Check sheet for the modelled part. Datum: model origin and axes. Units: mm. Face numbers are marked on the shaded views. Coordinates: 2 decimals unless noted, no trailing zeros. Write each loop counter-clockwise with the first axis right and the second up, starting at its lowest first coordinate (ties: lowest second). Pieces come first, ordered by that corner, then holes. Notation, with made-up numbers: (73, 12) -> (101, 12) arc R20 cw to (101, 31) -> close; hole circle Ø1 at (77.25, -11.5). An arc over 180 degrees is marked (long way). One line per item, written item: value. Start each with the question number.
1) Sectioned sample at C-C on y = -5.5. Enter the section's corners in (x, z), plus the area to 3 significant figures.
2) Sectioned sample at A-A on z = -6.75. Enter the section's corners in (x, y).
3) Sectioned sample at B-B on y = 2.25. Enter the section's corners in (x, z).
4) Scan lines: line 1 along Z through (x, y) = (-4.25, 5.5); line 2 along Y through (x, z) = (9.25, 5.25). Record each from-to range of solid material in increasing order. Write a range as [from, to].
5) Draft check along Y on the marked faces 1, 2 and 3. Enter one of: +Y half, -Y half, draft (parallel to the pull), parting line (faces both ways), or undercut.
6) Gauge pin test, flat end, axial feed: P1, Ø1, axis at x = -1.5, y = 2, coming from the +Z side. Record the tip position at first contact, or that the pin passes through.
7) Sectioned sample at D-D on z = 0.75. Enter the section's corners in (x, y).
Autodesk Inventor part; units mm, degrees
ref_plane "YZ Plane" through (0, 0, 0) normal (1, 0, 0) x (0, 1, 0)
ref_plane "XZ Plane" through (0, 0, 0) normal (0, 1, 0) x (-1, 0, 0)
ref_plane "XY Plane" through (0, 0, 0) normal (0, 0, 1) x (1, 0, 0)
sketch "Esboço1" plane through (0, 0, 0) normal (0, 0, 1) x (1, 0, 0)
  line L0 (-10, -10) -> (10, -10)
  line L1 (10, -10) -> (10, 10)
  line L2 (10, 10) -> (-10, 10)
  line L3 (-10, 10) -> (-10, -10)
  line L4 (-10, -10) -> (10, 10) construction
  line L5 (10, -10) -> (-10, 10) construction
  point P0 (0, 0)
  dimension "d0" = 20
  dimension "d1" = 20
extrude "Extrusão1" add sketch "Esboço1" along normal mid plane 20
sketch "Esboço2" plane through (0, 0, 10) normal (0, 0, 1) x (1, 0, 0)
  line L0 (-10, 10) -> (10, 10) construction
  line L1 (10, 10) -> (10, -10) construction
  line L2 (10, -10) -> (-10, -10) construction
  line L3 (-10, -10) -> (-10, 10) construction
  line L4 (5.9015, -7.5) -> (3.6163, -7.5)
  line L5 (3.6163, -7.5) -> (-0.0304, -1.5194)
  line L6 (-0.0304, -1.5194) -> (-3.75, -7.5)
  line L7 (-3.75, -7.5) -> (-5.9015, -7.5)
  line L8 (-5.9015, -7.5) -> (-1.1244, 0.0122)
  line L9 (-1.1244, 0.0122) -> (-5.7557, 7.5)
  line L10 (-5.7557, 7.5) -> (-3.4704, 7.5)
  line L11 (-3.4704, 7.5) -> (0.1033, 1.6288)
  line L12 (0.1033, 1.6288) -> (3.75, 7.5)
  line L13 (3.75, 7.5) -> (5.9015, 7.5)
  line L14 (5.9015, 7.5) -> (1.2095, 0.1094)
  line L15 (1.2095, 0.1094) -> (5.9015, -7.5)
  point P0 (0, 0)
extrude "Extrusão2" cut sketch "Esboço2" against normal blind 1
sketch "Esboço3" plane through (10, -10, 10) normal (1, 0, 0) x (0, 0, -1)
  line L0 (0, 20) -> (20, 20) construction
  line L1 (20, 20) -> (20, 0) construction
  line L2 (20, 0) -> (0, 0) construction
  line L3 (0, 0) -> (0, 20) construction
  line L4 (15.9562, 17.5) -> (10.8874, 9.137)
  line L5 (10.8874, 9.137) -> (10.8874, 2.5)
  line L6 (10.8874, 2.5) -> (8.8938, 2.5)
  line L7 (8.8938, 2.5) -> (8.8938, 8.9303)
  line L8 (8.8938, 8.9303) -> (3.825, 17.5)
  line L9 (3.825, 17.5) -> (6.0373, 17.5)
  line L10 (6.0373, 17.5) -> (9.9028, 10.8995)
  line L11 (9.9028, 10.8995) -> (13.8412, 17.5)
  line L12 (13.8412, 17.5) -> (15.9562, 17.5)
  point P0 (10, 10)
extrude "Extrusão3" cut sketch "Esboço3" against normal blind 1
sketch "Esboço4" plane through (-10, 10, 10) normal (0, 1, 0) x (1, 0, 0)
  line L0 (0, 20) -> (20, 20) construction
  line L1 (20, 20) -> (20, 0) construction
  line L2 (20, 0) -> (0, 0) construction
  line L3 (0, 0) -> (0, 20) construction
  line L4 (15.3181, 2.5) -> (4.84, 2.5)
  line L5 (4.84, 2.5) -> (4.84, 4.3598)
  line L6 (4.84, 4.3598) -> (12.8626, 15.7253)
  line L7 (12.8626, 15.7253) -> (5.2046, 15.7253)
  line L8 (5.2046, 15.7253) -> (5.2046, 17.5)
  line L9 (5.2046, 17.5) -> (15.1114, 17.5)
  line L10 (15.1114, 17.5) -> (15.1114, 15.701)
  line L11 (15.1114, 15.701) -> (7.0036, 4.2747)
  line L12 (7.0036, 4.2747) -> (15.3181, 4.2747)
  line L13 (15.3181, 4.2747) -> (15.3181, 2.5)
  point P0 (10, 10)
extrude "Extrusão4" cut sketch "Esboço4" against normal blind 1
properties part number "Cubo-0001-002" material "ABS plástico"
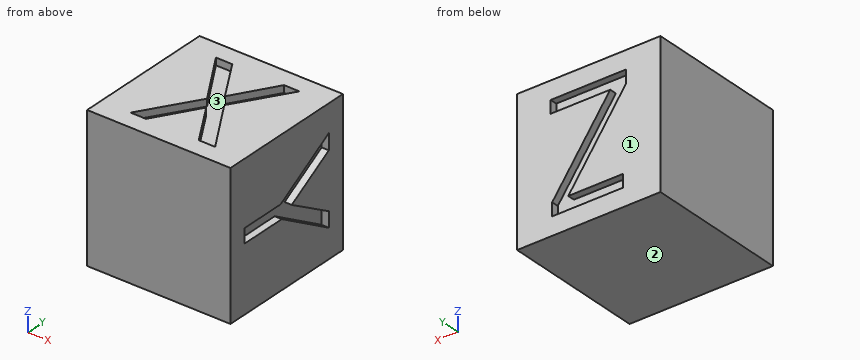
Answers:
1. outline: (-10, -10) -> (10, -10) -> (10, -0.89) -> (9, -0.89) -> (9, 1.11) -> (10, 1.11) -> (10, 10) -> (4.67, 10) -> (4.67, 9) -> (2.4, 9) -> (2.4, 10) -> (-2.51, 10) -> (-2.51, 9) -> (-4.63, 9) -> (-4.63, 10) -> (-10, 10) -> close
1. area: 394 mm2
2. outline: (-10, -10) -> (10, -10) -> (10, 10) -> (5.11, 10) -> (5.11, 9) -> (-4.8, 9) -> (-4.8, 10) -> (-10, 10) -> close
3. outline: (-10, -10) -> (10, -10) -> (10, -2.77) -> (9, -2.77) -> (9, -0.71) -> (10, -0.71) -> (10, 0.89) -> (9, 0.89) -> (9, 3.07) -> (10, 3.07) -> (10, 10) -> (2.57, 10) -> (2.57, 9) -> (0.49, 9) -> (0.49, 10) -> (-0.27, 10) -> (-0.27, 9) -> (-2.51, 9) -> (-2.51, 10) -> (-10, 10) -> close
4. line 1: z = [-10, 9]
4. line 2: y = [-10, 5.94], [7.5, 10]
5. face 1: +Y half
5. face 2: draft
5. face 3: undercut
6. P1: stops at z = 9
7. outline: (-10, -10) -> (10, -10) -> (10, -7.5) -> (9, -7.5) -> (9, 2.01) -> (10, 2.01) -> (10, 10) -> (0.53, 10) -> (0.53, 9) -> (-1.71, 9) -> (-1.71, 10) -> (-10, 10) -> close
